Geometry: final body of the model. Coordinates: model frame, mm. A direction names the side the tool comes from. Round coordinates to 2 decimals unless told otherwise and drop trailing zeros. Loops run counter-clockwise (first coordinate to the right, second up) from the corner with the lowest first, then second, coordinate; pieces in that order, holes last. Notation, with made-up numbers: (34.5, 44) - (44.5, 44) arc R23 ccw to (44.5, 79) - close; hole circle Ø6 at (-4, 43.25). An arc over 180 degrees is marked (long way). Answer as CSV lines item,"result".
from build123d import *

# Parameters (mm, degrees)
SKETCH1_W                = 6
SKETCH1_H                = 6
BOSS_EXTRUDE1_DEPTH      = 4
CUT_REVOLVE_THIN1_DEPTH  = 4
BOSS_EXTRUDE2_DEPTH      = 5.5
BOSS_EXTRUDE2_DEPTH_BACK = 5.5
SKETCH3_R                = 1
BOSS_EXTRUDE3_DEPTH      = 5.5
BOSS_EXTRUDE3_DEPTH_BACK = 5.5
SKETCH4_R                = 1


with BuildPart() as part:
    # Sketch1 → Boss-Extrude1 (new body)
    with BuildSketch(Plane(origin=(0, 0, 0), x_dir=(1, 0, 0), z_dir=(0, 1, 0))):
        Rectangle(SKETCH1_W, SKETCH1_H)
    extrude(amount=BOSS_EXTRUDE1_DEPTH)

    # Cut-Revolve-Thin1: read off the stored shape, not the designer's step
    # Cut-Revolve-Thin1 outline → Cut-Revolve-Thin1 (cut)
    with BuildSketch(Plane(origin=(0, 0, 0), x_dir=(1, 0, 0), z_dir=(0, 1, 0))):
        with BuildLine():
            ThreePointArc((3, -2.413514817), (2.722595616, -2.722595616), (2.413514817, -3))
            Line((2.413514817, -3), (3, -3))
            Line((3, -3), (3, -2.413514817))
        make_face()
        with BuildLine():
            Line((-3, -3), (-2.413514817, -3))
            ThreePointArc((-2.413514817, -3), (-2.722595616, -2.722595616), (-3, -2.413514817))
            Line((-3, -2.413514817), (-3, -3))
        make_face()
        with BuildLine():
            ThreePointArc((2.413514817, 3), (2.722595616, 2.722595616), (3, 2.413514817))
            Line((3, 2.413514817), (3, 3))
            Line((3, 3), (2.413514817, 3))
        make_face()
        with BuildLine():
            Line((-3, 3), (-3, 2.413514817))
            ThreePointArc((-3, 2.413514817), (-2.722595616, 2.722595616), (-2.413514817, 3))
            Line((-2.413514817, 3), (-3, 3))
        make_face()
    extrude(amount=CUT_REVOLVE_THIN1_DEPTH, mode=Mode.SUBTRACT)

    # Cut-Revolve-Thin1 2 outline → Cut-Revolve-Thin1 2 (revolve, cut)
    with BuildSketch(Plane.XY):
        Polygon((3.850331645, 4), (1.441154273, 4), (3.850331645, 2.609060796), align=None)
        Polygon((3.850331645, 0), (3.850331645, 1.390939204), (1.441154273, 0), align=None)
    revolve(axis=Axis((0, 0, 0), (0, 1, 0)), mode=Mode.SUBTRACT)

    # Sketch3 → Boss-Extrude2 (add, two sides: drawn at the far end of the back side and taken through both)
    with BuildSketch(Plane.XY.offset(-BOSS_EXTRUDE2_DEPTH_BACK)):
        with Locations((0, 2)):
            Circle(SKETCH3_R)
    extrude(amount=BOSS_EXTRUDE2_DEPTH + BOSS_EXTRUDE2_DEPTH_BACK)

    # Sketch4 → Boss-Extrude3 (add, two sides: drawn at the far end of the back side and taken through both)
    with BuildSketch(Plane(origin=(0, 0, 0), x_dir=(0, 0, -1), z_dir=(1, 0, 0)).offset(-BOSS_EXTRUDE3_DEPTH_BACK)):
        with Locations((0, 2)):
            Circle(SKETCH4_R)
    extrude(amount=BOSS_EXTRUDE3_DEPTH + BOSS_EXTRUDE3_DEPTH_BACK)


solid = part.part
(1) Section C-C (y = 2). Output: boundary loops of the cut face in (x, z), and give its area (3 significant figures).
Findings below:
outline,"(-5.5, -1) - (-3, -1) - (-3, -2.41) arc R3.85 ccw to (-2.41, -3) - (-1, -3) - (-1, -5.5) - (1, -5.5) - (1, -3) - (2.41, -3) arc R3.85 ccw to (3, -2.41) - (3, -1) - (5.5, -1) - (5.5, 1) - (3, 1) - (3, 2.41) arc R3.85 ccw to (2.41, 3) - (1, 3) - (1, 5.5) - (-1, 5.5) - (-1, 3) - (-2.41, 3) arc R3.85 ccw to (-3, 2.41) - (-3, 1) - (-5.5, 1) - close"
area,"55.4 mm2"
(2) Section A-A (z = 0). Output: boundary loops of the cut face in (x, y).
Findings below:
outline,"(-5.5, 1) - (-3, 1) - (-3, 0.9) - (-1.44, 0) - (1.44, 0) - (3, 0.9) - (3, 1) - (5.5, 1) - (5.5, 3) - (3, 3) - (3, 3.1) - (1.44, 4) - (-1.44, 4) - (-3, 3.1) - (-3, 3) - (-5.5, 3) - close"
(3) Material intervals for line 1 along Y through (x, z) = (0, 3.5); line 2 along Z through (x, y) = (-0.5, 2.95); line 3 along Y through (x, z) = (0.75, -1.25), sorted ascending.
Findings below:
line 1,"1 to 3"
line 2,"-3 to 3"
line 3,"0.01 to 3.99"
(4) Section B-B (x = 0). Output: boundary loops of the cut face in (y, z), and give its area (3 significant figures).
Findings below:
outline,"(0, -1.44) - (0.9, -3) - (1, -3) - (1, -5.5) - (3, -5.5) - (3, -3) - (3.1, -3) - (4, -1.44) - (4, 1.44) - (3.1, 3) - (3, 3) - (3, 5.5) - (1, 5.5) - (1, 3) - (0.9, 3) - (0, 1.44) - close"
area,"31.2 mm2"
(5) Pin query (flat end, axial travel): P1, Ø3, axis at x = 0.5, z = 3.5, coming from the -Y side; P2, Ø1.5, axis at y = 2, z = 3, coming from the -X side; P3, Ø1, axis at x = 0.5, z = 4.5, coming from the +Y side. Return the tip coordinate at first contact, or that it passes through.
Findings below:
P1,"y = 0.34"
P2,"x = -3"
P3,"y = 3"
(6) Access query for faces 1 (the face through (0, 1, 4)), 2 (the face through (0, 1, -4)), 3 (the face through (-4, 1, 0)), 4 (the face through (4, 1, 0)), 5 (the face through (0, 2, 5.5)). Directions: +Z, -Z, +X, -X, +Y, -Y. A direction counts if a zero-diameter tool reaches every point of the face in a straight line with its end or side. Return the directions, or none.
Findings below:
face 1,"+Z"
face 2,"-Z"
face 3,"-X"
face 4,"+X"
face 5,"+Z, +X, -X, +Y, -Y"
(7) Section D-D (z = 4). Output: boundary loops of the cut face in (x, y), and give its area (3 significant figures).
Findings below:
outline,"circle Ø2 at (0, 2)"
area,"3.14 mm2"
